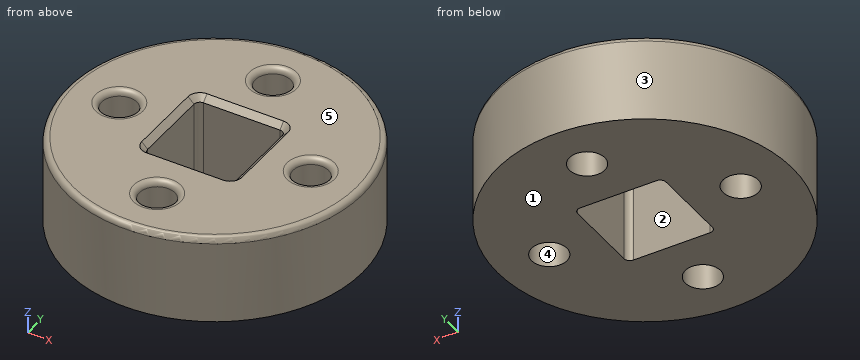
```python
from build123d import *

# Parameters (mm, degrees)
F0_R     = 25
F1_DEPTH = 15
F2_R     = 3
F3_DEPTH = 15
F4_R     = 1
F5_SIZE  = 1


with BuildPart() as f1:
    # F0 (on Top) → F1 (new body)
    with BuildSketch(Plane.XY):
        with Locations((-0.018229, 0.1201)):
            Circle(F0_R)
        with BuildLine():
            Line((6.481771, -7.3799), (-6.518229, -7.3799))
            ThreePointArc((-6.518229, -7.3799), (-7.225335, -7.087007), (-7.518229, -6.3799))
            Line((-7.518229, -6.3799), (-7.518229, 6.6201))
            ThreePointArc((-7.518229, 6.6201), (-7.225335, 7.327207), (-6.518229, 7.6201))
            Line((-6.518229, 7.6201), (6.481771, 7.6201))
            ThreePointArc((6.481771, 7.6201), (7.188878, 7.327207), (7.481771, 6.6201))
            Line((7.481771, 6.6201), (7.481771, -6.3799))
            ThreePointArc((7.481771, -6.3799), (7.188878, -7.087007), (6.481771, -7.3799))
        make_face(mode=Mode.SUBTRACT)
    extrude(amount=F1_DEPTH)

    # F2 (on face) → F3 (cut)
    with BuildSketch(Plane.XY.offset(15)):
        with Locations((-0.018229, -16.1299)):
            Circle(F2_R)
        with Locations((16.231771, 0.1201)):
            Circle(F2_R)
        with Locations((-0.018229, 16.3701)):
            Circle(F2_R)
        with Locations((-16.268229, 0.1201)):
            Circle(F2_R)
    extrude(amount=-F3_DEPTH, mode=Mode.SUBTRACT)

    # F4
    f4_edges = [f1.edges().sort_by_distance(p)[0] for p in [
        (-25.018229, 0.1201, 15),
        (-19.268229, 0.1201, 15),
        (-3.018229, 16.3701, 15),
        (-3.018229, -16.1299, 15),
        (13.231771, 0.1201, 15),
    ]]
    fillet(f4_edges, radius=F4_R)

    # F5
    f5_edges = [f1.edges().sort_by_distance(p)[0] for p in [
        (-0.018229, -7.3799, 15),
        (7.481771, 0.1201, 15),
        (-0.018229, 7.6201, 15),
        (-7.518229, 0.1201, 15),
    ]]
    chamfer(f5_edges, length=F5_SIZE)


solid = f1.part
```
Design review of the part built by this model. Coordinates are the model's own, in mm. Face numbers are marked on the shaded views. A direction names the side the tool comes from. Give positions to 0.01 mm unless a question says otherwise; leave off trailing zeros. Order: outer loops, then holes, each group sorted by start corner. A loop starts at its lowest first (then second) coordinate and runs counter-clockwise, first axis right, second up. Notation, with made-up numbers: (21, 65) -> (63, 65) arc R13 cw to (63, 86) -> close; hole circle Ø5 at (38.5, 8.5). An arc over 180 degrees is marked (long way). Write item = value, one per line. Start each with the question number.
(1) We need section A-A on z = 7.75. Write out the cut boundary in (x, y), plus the area to 3 significant figures.
(2) To check wall thickness, follow line 1 along Y through (x, z) = (-1.5, 11.75); line 2 along X through (y, z) = (-2, 6); line 3 along Y through (x, z) = (-15, 1.75). State the ranges of each line that lie inside material, in increasing order.
(3) Mouldability with a two-part tool opening along X and no side actions: class the marked faces 3, 4 and 5 as +X half, -X half, draft (parallel to the pull), parting line (faces both ways), or undercut.
(4) We need section B-B on y = -0.5. State how many separate pieces and enclosed holes the cut face has, plus the area to 3 significant figures.
(5) For pin 1 (4 mm diameter, centred on x = 0, z = 9.5, fed in from -Y); pin 2 (5 mm diameter, centred on x = -4.5, z = 12.5, fed in from +Y); pin 3 (8 mm diameter, centred on y = 9.5, z = 12, fed in from -X); pin 4 (5.5 mm diameter, centred on x = -0.02, y = -16.13, fed in from -Z), all flat-tipped, find the tip position at first contact; note any pin that passes through.
(6) For the marked faces 1 and 2, list the 3-axis set-ups (+Z, -Z, +X, -X, +Y, -Y) from which the entire face can be reached by the end or side of a thin tool; tool diameter is ignored.
Numbers:
q1.outline = circle Ø50 at (-0.02, 0.12); hole circle Ø6 at (-16.27, 0.12); hole (-7.52, -6.38) arc R1 ccw to (-6.52, -7.38) -> (6.48, -7.38) arc R1 ccw to (7.48, -6.38) -> (7.48, 6.62) arc R1 ccw to (6.48, 7.62) -> (-6.52, 7.62) arc R1 ccw to (-7.52, 6.62) -> close; hole circle Ø6 at (-0.02, -16.13); hole circle Ø6 at (-0.02, 16.37); hole circle Ø6 at (16.23, 0.12)
q1.area = 1,630 mm^2
q2.line_1 = -24.84 to -18.74, -13.52 to -7.38, 7.62 to 13.76, 18.98 to 25.08
q2.line_2 = -24.93 to -18.39, -14.15 to -7.52, 7.48 to 14.11, 18.35 to 24.89
q2.line_3 = -19.89 to -2.6, 2.84 to 20.13
q3.face_3 = parting line
q3.face_4 = undercut
q3.face_5 = draft
q4.separate_pieces = 4
q4.enclosed_holes = 0
q4.area = 346 mm^2
q5.pin_1 = -24.88
q5.pin_2 = 25.04
q5.pin_3 = -24.43
q5.pin_4 = through
q6.face_1 = -Z, +X, -X, +Y, -Y
q6.face_2 = +Z, -Z
